Here's how the part is built. I have some questions about the finished solid (model axes, mm). Face numbers are marked on the shaded views. A direction names the side the tool comes from. Coordinates: 2 decimals unless noted, no trailing zeros. Loops run counter-clockwise (first coordinate to the right, second up) from the corner with the lowest first, then second, coordinate; pieces in that order, holes last. Notation, with made-up numbers: (38, 64.5) -> (78, 64.5) arc R34 cw to (78, 102.5) -> close; hole circle Ø9 at (17, 43). An arc over 180 degrees is marked (long way). Answer as a JSON object with one key per item and string values. Group by question number.
Q1. I want a section at B-B on y = 0. Write out the boundary of the cut face in (x, z).
Q2. I want a section at A-A on x = 0. Write out the boundary of the cut face in (y, z).
Q3. I want a section at C-C on z = -4. Write out the boundary of the cut face in (x, y).
Q4. I want a section at D-D on y = -7.25. Write out the boundary of the cut face in (x, z).
Q5. On a 3-axis mill with a long thin cutter (end or side, diameter ignored), from which of +Z, -Z, +X, -X, +Y, -Y can I reach the whole of each face in a straight line? I mean the marked faces 1, 2 and 3. Say none if no direction works.
Q6. I need wall thicknesses on line 1 (Y direction, x = 0, z = -3.95); line 2 (Y direction, x = 0, z = -0.8); line 3 (Z direction, x = 7, y = -6). Which ranges of each line are inside material? Lowest first, please.
Q7. I'm going to push flat-ended pins straight in: pin 1 (1 mm diameter, centred on x = 3.5, z = -7.5, fed in from +Y); pin 2 (1.5 mm diameter, centred on x = 8.5, z = -2.5, fed in from -Y); pin 3 (1.5 mm diameter, centred on x = -3, z = -1.5, fed in from -Y); pin 4 (12 mm diameter, centred on x = 0, y = 0, fed in from +Z). Where does each tip first touch, or does it pass through?
Q8. Thinking about a two-plate mould opening in Y: for the marked faces 4, 5, 6 and 7, which applies, released by +Y, released by -Y, zero draft, split by the parting line, or undercut?
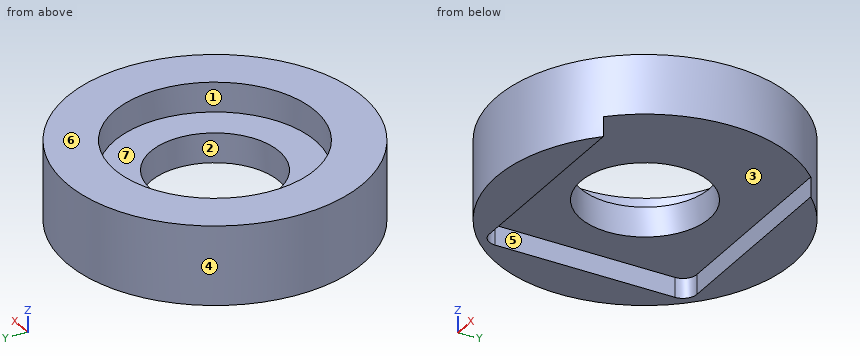
Autodesk Inventor part; units mm, degrees
ref_plane "YZ Plane" through (0, 0, 0) normal (1, 0, 0) x (0, 1, 0)
ref_plane "XZ Plane" through (0, 0, 0) normal (0, 1, 0) x (-1, 0, 0)
ref_plane "XY Plane" through (0, 0, 0) normal (0, 0, 1) x (1, 0, 0)
sketch "Sketch8" plane through (0, 0, 0) normal (0, 0, 1) x (1, 0, 0)
  circle A0 centre (0, 0) radius 15
  dimension "d33" = 30
extrude "Extrusion7" add sketch "Sketch8" against normal blind 8
sketch "Sketch10" plane through (0, 0, -8) normal (0, 0, -1) x (-1, 0, 0)
  line L0 (9, 10.07) -> (-29.1, 10.07)
  arc A0 (10, 9.07) -> (9, 10.07) centre (9, 9.07) ccw
  line L1 (10, 9.07) -> (10, -9.07)
  arc A1 (9, -10.07) -> (10, -9.07) centre (9, -9.07) ccw
  line L2 (-29.1, -10.07) -> (9, -10.07)
  line L3 (-29.1, 10.07) -> (-29.1, -10.07)
  arc A2 (9, -10.47) -> (10.4, -9.07) centre (9, -9.07) ccw
  line L4 (10.4, -9.07) -> (10.4, 9.07)
  arc A3 (10.4, 9.07) -> (9, 10.47) centre (9, 9.07) ccw
  line L5 (9, 10.47) -> (-29.5, 10.47)
  line L6 (-29.5, 10.47) -> (-29.5, -10.47)
  line L7 (-29.5, -10.47) -> (9, -10.47)
  dimension "d59" = 0.4
extrude "Extrusion8" cut sketch "Sketch10" against normal blind 2 contours A0 L1 A1 L2 L3 L0 | L7 L6 L5 A3 L4 A2
sketch "Sketch11" plane through (0, 0, -6) normal (0, 0, -1) x (-1, 0, 0)
  circle A0 centre (0, 0) radius 6.4
  circle A1 centre (0, 0) radius 6.5
  point P0 (0, 0)
  dimension "d58" = 13
extrude "Extrusion9" cut sketch "Sketch11" against normal through all contours A0 | A1
sketch "Sketch13" plane through (0, 0, 0) normal (0, 0, 1) x (1, 0, 0)
  circle A0 centre (0, 0) radius 9.96
  circle A1 centre (0, 0) radius 10.16
  point P0 (0, 0)
  dimension "d44" = 0.2
extrude "Extrusion11" cut sketch "Sketch13" against normal blind 3 contours A0 | A1
properties part number "axis_19_bottom_frame" material "Aluminum 6061-AHC"
Result set:
{
 "1": {"outline": "(-15, -8) -> (-10.4, -8) -> (-10.4, -6) -> (-6.5, -6) -> (-6.5, -3) -> (-10.16, -3) -> (-10.16, 0) -> (-15, 0) -> close; (6.5, -6) -> (15, -6) -> (15, 0) -> (10.16, 0) -> (10.16, -3) -> (6.5, -3) -> close"},
 "2": {"outline": "(-15, -8) -> (-10.47, -8) -> (-10.47, -6) -> (-6.5, -6) -> (-6.5, -3) -> (-10.16, -3) -> (-10.16, 0) -> (-15, 0) -> close; (6.5, -6) -> (10.47, -6) -> (10.47, -8) -> (15, -8) -> (15, 0) -> (10.16, 0) -> (10.16, -3) -> (6.5, -3) -> close"},
 "3": {"outline": "circle Ø30 at (0, 0); hole circle Ø13 at (0, 0)"},
 "4": {"outline": "(-13.13, -8) -> (-10.4, -8) -> (-10.4, -6) -> (13.13, -6) -> (13.13, 0) -> (7.12, 0) -> (7.12, -3) -> (-7.12, -3) -> (-7.12, 0) -> (-13.13, 0) -> close"},
 "5": {"face 1": "+Z", "face 2": "+Z, -Z", "face 3": "-Z, +X"},
 "6": {"line 1": "y = -15 to -6.5, 6.5 to 15", "line 2": "y = -15 to -10.16, 10.16 to 15", "line 3": "z = -6 to -3"},
 "7": {"pin 1": "stops at y = 14.7", "pin 2": "stops at y = -12.84", "pin 3": "stops at y = -14.83", "pin 4": "passes through"},
 "8": {"face 4": "split by the parting line", "face 5": "undercut", "face 6": "zero draft", "face 7": "undercut"}
}
